Check sheet for the modelled part. Datum: model origin and axes. Units: mm. Face numbers are marked on the shaded views. A direction names the side the tool comes from. Give positions to 0.01 mm unless a question says otherwise; leave off trailing zeros. Order: outer loops, then holes, each group sorted by start corner. A loop starts at its lowest first (then second) coordinate and runs counter-clockwise, first axis right, second up.
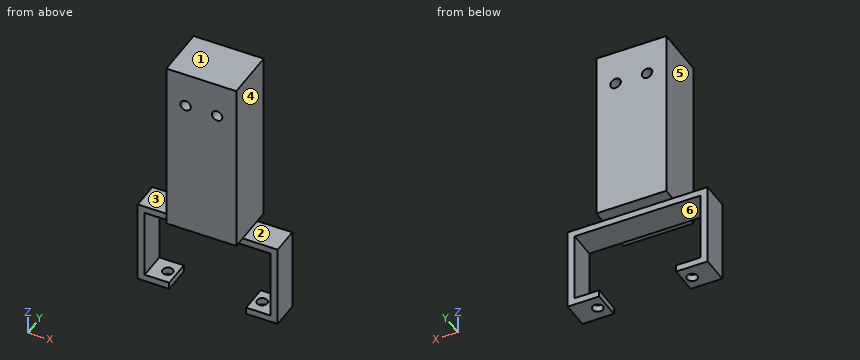
```python
from build123d import *

# Parameters (mm, degrees)
SKETCH_8_W          = 9
SKETCH_8_H          = 8
SKETCH_8_R          = 1.5
EXTRUDE_1_DEPTH     = 2
EXTRUDE_1_2_DEPTH   = 2
SKETCH_9_W          = 2
SKETCH_9_H          = 8
EXTRUDE_2_DEPTH     = 20
SKETCH_10_W         = 40
SKETCH_10_H         = 8
EXTRUDE_3_DEPTH     = 2
SKETCH_11_W         = 20
SKETCH_11_H         = 15
EXTRUDE_4_DEPTH     = 50
SKETCH_12_R         = 1.5
CUT_EXTRUDE_1_DEPTH = 79.108898341


with BuildPart() as part:
    # Sketch 8 → Extrude 1 (new body)
    with BuildSketch(Plane.XY):
        with Locations((-15.5, 0)):
            Rectangle(SKETCH_8_W, SKETCH_8_H)
        with Locations((-13.5, 0)):
            Circle(SKETCH_8_R, mode=Mode.SUBTRACT)
    extrude(amount=EXTRUDE_1_DEPTH)



with BuildPart() as body_2:
    # Sketch 8 → Extrude 1 2 (new body)
    with BuildSketch(Plane.XY):
        with Locations((15.5, 0)):
            Rectangle(SKETCH_8_W, SKETCH_8_H)
        with Locations((13.5, 0)):
            Circle(SKETCH_8_R, mode=Mode.SUBTRACT)
    extrude(amount=EXTRUDE_1_2_DEPTH)


with BuildPart() as part_1:
    add(part.part)

    add(body_2.part)  # Extrude 2 merges body 2
    # Sketch 9 → Extrude 2 (add)
    with BuildSketch(Plane.XY.offset(2)):
        with Locations((-19, 0)):
            Rectangle(SKETCH_9_W, SKETCH_9_H)
        with Locations((19, 0)):
            Rectangle(SKETCH_9_W, SKETCH_9_H)
    extrude(amount=EXTRUDE_2_DEPTH)

    # Sketch 10 → Extrude 3 (add)
    with BuildSketch(Plane.XY.offset(22)):
        Rectangle(SKETCH_10_W, SKETCH_10_H)
    extrude(amount=EXTRUDE_3_DEPTH)

    # Sketch 11 → Extrude 4 (add)
    with BuildSketch(Plane.XY.offset(24)):
        Rectangle(SKETCH_11_W, SKETCH_11_H)
    extrude(amount=EXTRUDE_4_DEPTH)

    # Sketch 12 → Cut-Extrude 1 (cut, through all)
    with BuildSketch(Plane(origin=(0, 7.5, 0), x_dir=(1, 0, 0), z_dir=(0, 1, 0))):
        with Locations(Location((-4.5, -64, 0), (0, 0, 270))):
            Circle(SKETCH_12_R)
        with Locations(Location((4.5, -64, 0), (0, 0, 270))):
            Circle(SKETCH_12_R)
    extrude(amount=-CUT_EXTRUDE_1_DEPTH, mode=Mode.SUBTRACT)


solid = part_1.part
```
(1) Cross-section at B-B on x = 4.5. Enter the section's corners in (y, z).
Response values:
outline: (-7.5, 24) - (-4, 24) - (-4, 22) - (4, 22) - (4, 24) - (7.5, 24) - (7.5, 62.5) - (-7.5, 62.5) - close; (-7.5, 65.5) - (7.5, 65.5) - (7.5, 74) - (-7.5, 74) - close
(2) Cross-section at D-D on z = 64. Enter the section's corners in (x, y), then the cut area to 3 significant figures.
Response values:
outline: (-10, -7.5) - (-6, -7.5) - (-6, 7.5) - (-10, 7.5) - close; (-3, -7.5) - (3, -7.5) - (3, 7.5) - (-3, 7.5) - close; (6, -7.5) - (10, -7.5) - (10, 7.5) - (6, 7.5) - close
area: 210 mm2
(3) Cross-section at C-C on z = 12. Enter the section's corners in (x, y).
Response values:
outline: (-20, -4) - (-18, -4) - (-18, 4) - (-20, 4) - close; (18, -4) - (20, -4) - (20, 4) - (18, 4) - close
(4) Release check for a two-part mould opening along X. For the marked faces 3, 4, 5 and 6 record: released by +X, released by -X, zero draft, split by the parting line, or undercut.
Response values:
face 3: zero draft
face 4: released by +X
face 5: released by -X
face 6: undercut
(5) Material ranges on L1, parallel to X at y = -3.5, z = 64; L2, parallel to X at y = -3.25, z = 6.5; L3, parallel to Z at x = 11.5, y = 3.25, recorded low to high.
Response values:
L1: x = -10 to -6, -3 to 3, 6 to 10
L2: x = -20 to -18, 18 to 20
L3: z = 0 to 2, 22 to 24
(6) Cross-section at A-A on y = 0. Enter the section's corners in (x, z).
Response values:
outline: (-20, 0) - (-15, 0) - (-15, 2) - (-18, 2) - (-18, 22) - (18, 22) - (18, 2) - (15, 2) - (15, 0) - (20, 0) - (20, 24) - (10, 24) - (10, 74) - (-10, 74) - (-10, 24) - (-20, 24) - close; (-12, 0) - (-11, 0) - (-11, 2) - (-12, 2) - close; (11, 0) - (12, 0) - (12, 2) - (11, 2) - close; hole circle Ø3 at (-4.5, 64); hole circle Ø3 at (4.5, 64)
(7) Gauge pin test, flat ends, axial feed: pin 1 Ø6.5 at (x, y) = (-1, 1.5) entering from -Z; pin 2 Ø2 at (x, y) = (-13.5, -0.5) entering from +Z; pin 3 Ø4 at (x, y) = (3, -6.5) entering from -Z. Record the tip position at first contact, or that the pin passes through.
Response values:
pin 1: stops at z = 22
pin 2: stops at z = 24
pin 3: stops at z = 24
(8) Set-up check for the marked faces 1 and 2: record each of +Z, -Z, +X, -X, +Y, -Y from which the full face is reachable in a straight line by a thin tool's end or side.
Response values:
face 1: +Z, +X, -X, +Y, -Y
face 2: +Z, +X, +Y, -Y
